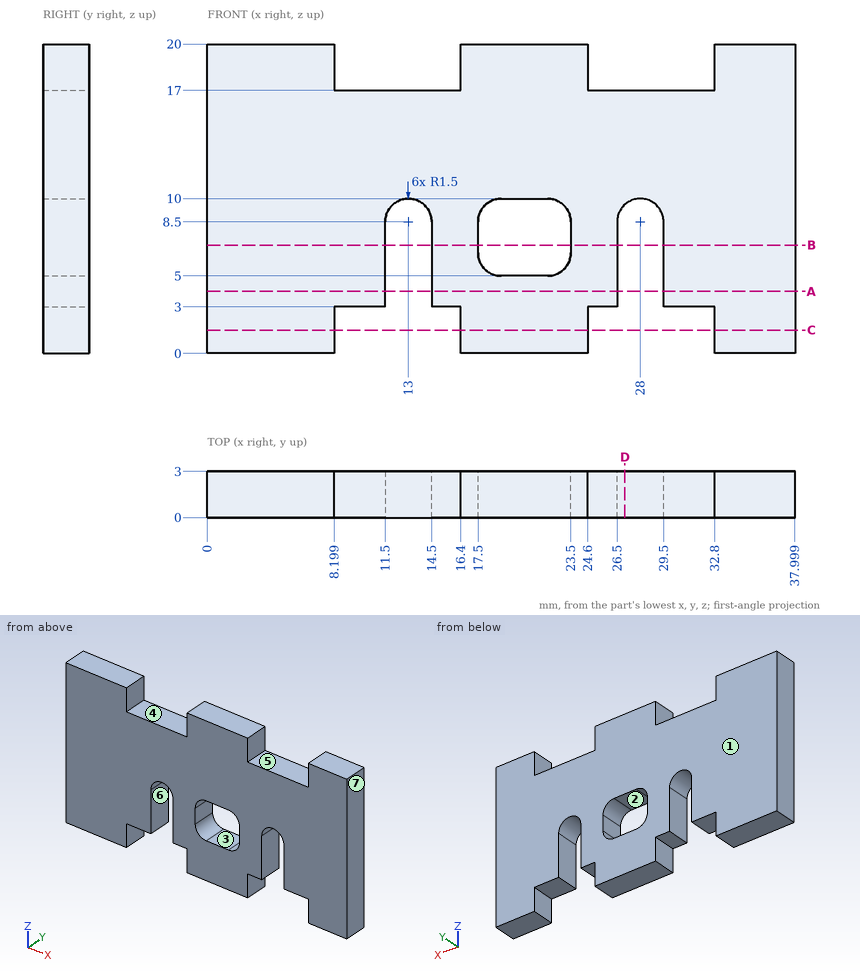
Answer from the drawing. Dimensions are ordinates in mm from the lowest x, y and z of the part. A direction names the side the tool comes from. Round coordinates to 2 decimals unless told otherwise and drop trailing zeros. Write each loop counter-clockwise with the first axis right and the second up, starting at its lowest first coordinate (ties: lowest second). Pieces come first, ordered by that corner, then holes. Notation, with made-up numbers: M 36,-35 L 52,-35 A33 cw 52,3 Z; hole C 23,-26.5 d8. An arc over 180 degrees is marked long. One line per item, written item: value.
Q1. Find section B-B on z = 7. Write down the section's boundary in (x, y).
Data:
outline: M 0,0 L 11.5,0 L 11.5,3 L 0,3 Z; M 14.5,0 L 17.5,0 L 17.5,3 L 14.5,3 Z; M 23.5,0 L 26.5,0 L 26.5,3 L 23.5,3 Z; M 29.5,0 L 38,0 L 38,3 L 29.5,3 Z
Q2. Find section C-C on z = 1.5. Write down the section's boundary in (x, y).
Data:
outline: M 0,0 L 8.2,0 L 8.2,3 L 0,3 Z; M 16.4,0 L 24.6,0 L 24.6,3 L 16.4,3 Z; M 32.8,0 L 38,0 L 38,3 L 32.8,3 Z
Q3. Find section A-A on z = 4. Write down the section's boundary in (x, y).
Data:
outline: M 0,0 L 11.5,0 L 11.5,3 L 0,3 Z; M 14.5,0 L 26.5,0 L 26.5,3 L 14.5,3 Z; M 29.5,0 L 38,0 L 38,3 L 29.5,3 Z
Q4. Straight lines are drawn through the part: line 1 (X direction, y = 2.2, z = 7.5); line 2 (X direction, y = 1.35, z = 3.5); line 3 (X direction, y = 2.5, z = 18.5). For each, find the intervals that lie inside material, in ascending order. Write a range as [from, to].
Data:
line 1: [0, 11.5], [14.5, 17.5], [23.5, 26.5], [29.5, 38]
line 2: [0, 11.5], [14.5, 26.5], [29.5, 38]
line 3: [0, 8.2], [16.4, 24.6], [32.8, 38]
Q5. For a pull along Z with two mould halves and no side action, classify the marked faces 1, 2, 3 and 4 as +Z half, -Z half, draft (parallel to the pull), parting line (faces both ways), or undercut.
Data:
face 1: draft
face 2: undercut
face 3: undercut
face 4: +Z half
Q6. Which of the six approach directions +Z, -Z, +X, -X, +Y, -Y give full straight-line access (tool end or side, diameter ignored) to the marked faces 5, 6 and 7?
Data:
face 5: +Z, +Y, -Y
face 6: -Z, +Y, -Y
face 7: +Z, -Z, +X, +Y, -Y
Q7. Flat-ended cylindrical pins translate along their axes: pin 1 Ø1.5 at (x, y) = (11, 1.5) entering from +Z; pin 2 Ø0.9 at (x, y) = (10.5, 2) entering from -Z. Find the tip coordinate at first contact, or state that the pin passes through.
Data:
pin 1: z = 17
pin 2: z = 3
Q8. Find section D-D on x = 27. Write down the section's boundary in (y, z).
Data:
outline: M 0,9.62 L 3,9.62 L 3,17 L 0,17 Z
